from build123d import *

# Parameters (mm, degrees)
SKETCH2_W          = 57.15
SKETCH2_H          = 31.75
BASE_FLANGE1_DEPTH = 3.175
EDGE_FLANGE1_DEPTH = 31.75
CUT_EXTRUDE1_DEPTH = 3.175


# Sheet-metal steps are written as plain solids
with BuildPart() as part:
    # Sketch2 → Base-Flange1 (new body)
    with BuildSketch(Plane.XY):
        Rectangle(SKETCH2_W, SKETCH2_H)
    extrude(amount=BASE_FLANGE1_DEPTH)

    # Edge-Flange1 section (across the edge) → Edge-Flange1 (add)
    with BuildSketch(Plane(origin=(29.575, -15.875, 3.175), x_dir=(-1, 0, 0), z_dir=(0, 1, 0))):
        with BuildLine():
            Line((-3.175, 1), (-3.175, 41.275))
            Line((-3.175, 41.275), (0, 41.275))
            Line((0, 41.275), (0, 1))
            ThreePointArc((0, 1), (0.292893219, 0.292893219), (1, 0))
            Line((1, 0), (1, -3.175))
            ThreePointArc((1, -3.175), (-1.952170811, -1.952170811), (-3.175, 1))
        make_face()
    extrude(amount=EDGE_FLANGE1_DEPTH)

    # Sketch10 → Cut-Extrude1 (cut)
    with BuildSketch(Plane(origin=(32.75, 0, 0), x_dir=(0, 0, -1), z_dir=(1, 0, 0))):
        Polygon((-4.175, 15.875), (-44.45, -15.875), (-44.45, 15.875), align=None)
    extrude(amount=-CUT_EXTRUDE1_DEPTH, mode=Mode.SUBTRACT)


solid = part.part
The listing builds one solid part. Answer for the finished solid, in the listing's coordinates (mm). A direction names the side the tool comes from. Coordinates: 2 decimals unless noted, no trailing zeros. Loops run counter-clockwise (first coordinate to the right, second up) from the corner with the lowest first, then second, coordinate; pieces in that order, holes last.
1) Find the intervals of material crossed by L1, parallel to Z at x = 19, y = 9 (3 decimals); L2, parallel to X at y = -12.5, z = 32 (3 decimals); L3, parallel to X at y = 9.5, z = 4, in increasing order.
2) Find section D-D on y = -13. Write down the section's boundary in (x, z) (3 decimals).
3) Determine the mould class of faces 1 (the face through (11, -15.875, 3)), 2 (the face through (2, 15.875, 2)), 3 (the face through (0, 0, 0)) for opening direction Y: pulls with the +Y half, pulls with the -Y half, needs draft (parallel to the pull), parting line crosses it, or undercut.
4) A tool of negligible diameter and unlimited length cuts with its end or side. For faces 4 (the face through (-28.575, 0, 2)), 5 (the face through (29.575, -7, 16)), from which of +Z, -Z, +X, -X, +Y, -Y can it reach the whole face along a straight path? Write none if from no direction.
5) Find section C-C on z = 35. Write down the section's boundary in (x, y) (3 decimals), then the cut area to 3 significant figures.
6) Find section B-B on y = -7.5. Write down the section's boundary in (x, z) (3 decimals), then the cut area to 3 significant figures.
7) A flat-ended cylindrical pin translates along its axis: pin 1 Ø6 at (y, z) = (-4.5, 15) entering from -X (3 decimals). Find the tip coordinate at first contact, or state that the pin passes through.
8) Find section A-A on x = -13. Write down the section's boundary in (y, z) (3 decimals), then the cut area to 3 significant figures.
Values:
1. L1: z = 0 to 3.175
1. L2: x = 29.575 to 32.75
1. L3: x = 29.56 to 32.75
2. outline: (-28.575, 0) - (28.575, 0) arc R4.175 ccw to (32.75, 4.175) - (32.75, 40.803) - (29.575, 40.803) - (29.575, 4.175) arc R1 cw to (28.575, 3.175) - (-28.575, 3.175) - close
3. face 1: pulls with the -Y half
3. face 2: pulls with the +Y half
3. face 3: needs draft
4. face 4: +Z, -Z, -X, +Y, -Y
4. face 5: +Z, -X, +Y, -Y
5. outline: (29.575, -15.875) - (32.75, -15.875) - (32.75, -8.425) - (29.575, -8.425) - close
5. area: 23.7 mm2
6. outline: (-28.575, 0) - (28.575, 0) arc R4.175 ccw to (32.75, 4.175) - (32.75, 33.826) - (29.575, 33.826) - (29.575, 4.175) arc R1 cw to (28.575, 3.175) - (-28.575, 3.175) - close
6. area: 288 mm2
7. pin 1: stops at x = 29.575
8. outline: (-15.875, 0) - (15.875, 0) - (15.875, 3.175) - (-15.875, 3.175) - close
8. area: 101 mm2
